The model under review builds one solid part; all positions refer to its coordinate system, in mm. Face numbers are marked on the shaded views. A direction names the side the tool comes from. Give positions to 0.01 mm unless a question says otherwise; leave off trailing zeros. Write each loop counter-clockwise with the first axis right and the second up, starting at its lowest first coordinate (ties: lowest second). Pieces come first, ordered by that corner, then holes.
from build123d import *

# Parameters (mm, degrees)
SKETCH1_W               = 101.6
SKETCH1_H               = 85.471
BOSS_EXTRUDE1_DEPTH     = 1.6002
SKETCH2_W               = 21.717
SKETCH2_H               = 16.002
ETHERNET_DEPTH          = 14.224
SKETCH3_W               = 13.9192
SKETCH3_H               = 8.89
POWER_CONNECTOR_DEPTH   = 10.6172
SKETCH4_W               = 9.0424
SKETCH4_H               = 32.9438
SKETCH4_H_2             = 20.2184
F_2X_CONNECTOR_DEPTH    = 9.2456
SKETCH6_W               = 15.24
SKETCH6_H               = 13.716
SD_CARD_DEPTH           = 2.3876
SKETCH7_R               = 5.08
CAPACATOR_DEPTH         = 16.9164
SKETCH5_R               = 1.6891
CORNER_HOLE_DEPTH       = 71.754645263
MIRROR2_COPY_1_SKETCH_R = 1.6891
MIRROR2_COPY_1_DEPTH    = 71.754645263


with BuildPart() as part:
    # Sketch1 → Boss-Extrude1 (new body)
    with BuildSketch(Plane.XY):
        Rectangle(SKETCH1_W, SKETCH1_H)
    extrude(amount=BOSS_EXTRUDE1_DEPTH)

    # Sketch2 → Ethernet (add)
    with BuildSketch(Plane.XY.offset(1.6002)):
        with Locations((-39.9415, 11.8745)):
            Rectangle(SKETCH2_W, SKETCH2_H)
    extrude(amount=ETHERNET_DEPTH)

    # Sketch3 → Power Connector (add)
    with BuildSketch(Plane.XY.offset(1.6002)):
        with Locations((-46.2534, -30.4165)):
            Rectangle(SKETCH3_W, SKETCH3_H)
    extrude(amount=POWER_CONNECTOR_DEPTH)

    # Sketch4 → 2x Connector (add)
    with BuildSketch(Plane.XY.offset(1.6002)):
        with Locations((48.7426, 12.954)):
            Rectangle(SKETCH4_W, SKETCH4_H)
        with Locations((48.7426, -13.6779)):
            Rectangle(SKETCH4_W, SKETCH4_H_2)
    extrude(amount=F_2X_CONNECTOR_DEPTH)

    # Sketch6 → SD Card (add)
    with BuildSketch(Plane.XY.offset(1.6002)):
        with Locations((-42.291, 28.8925)):
            Rectangle(SKETCH6_W, SKETCH6_H)
    extrude(amount=SD_CARD_DEPTH)

    # Sketch7 → Capacator (add)
    with BuildSketch(Plane.XY.offset(1.6002)):
        with Locations(Location((-26.797, -28.2575, 0), (0, 0, 180))):
            Circle(SKETCH7_R)
    extrude(amount=CAPACATOR_DEPTH)

    # Sketch5 → Corner Hole (cut, through all)
    with BuildSketch(Plane(origin=(0, 0, 0), x_dir=(-1, 0, 0), z_dir=(0, 0, -1))):
        with Locations((-47.3329, 39.4462)):
            Circle(SKETCH5_R)
    corner_hole = extrude(amount=-CORNER_HOLE_DEPTH, mode=Mode.SUBTRACT)

    # Mirror1: Corner Hole across plane
    add(corner_hole.mirror(Plane(origin=(0, 0, 0), x_dir=(0, 0, 1), z_dir=(1, 0, 0))), mode=Mode.SUBTRACT)

    # Mirror2: Corner Hole across plane
    add(corner_hole.mirror(Plane.ZX), mode=Mode.SUBTRACT)

    # Mirror2 copy 1 sketch → Mirror2 copy 1 (cut, through all)
    with BuildSketch(Plane(origin=(0, 0, 0), x_dir=(1, 0, 0), z_dir=(0, 0, -1))):
        with Locations((-47.3329, 39.4462)):
            Circle(MIRROR2_COPY_1_SKETCH_R)
    extrude(amount=-MIRROR2_COPY_1_DEPTH, mode=Mode.SUBTRACT)


solid = part.part
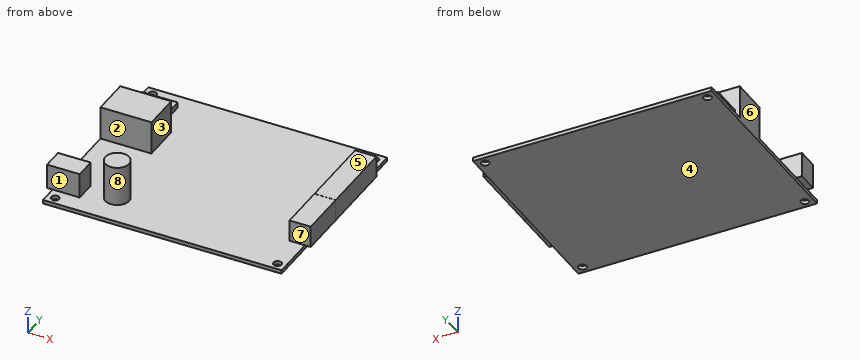
1) Consider section B-B, the plane y = -15. Give the boundary of the cut face in (x, z), then the cut area to 3 significant figures.
2) Consider section D-D, the plane y = 17. Give the boundary of the cut face in (x, z).
3) To check wall thickness, follow probe 1 along X at (y, z) = (9, 2.25); probe 2 along Y at (x, z) = (-43, 12); probe 3 along X at (y, z) = (-18, 9.5). State the ranges of each line that lie inside material, in increasing order.
4) Consider section A-A, the plane x = -38. Give the boundary of the cut face in (y, z).
5) Consider section C-C, the plane z = 9.5. Give the boundary of the cut face in (x, y).
6) The part is to be moulded in two halves that separate along X. For the marked faces 6, 7 and 8, say which applies: +X half, -X half, draft (parallel to the pull), parting line (faces both ways), or undercut.
7) Insertion check: pin 1 (1 mm diameter, centred on x = -8.5, y = -1, fed in from +Z); pin 2 (2.5 mm diameter, centred on y = 26.5, z = 2.5, fed in from -X); pin 3 (0.7 mm diameter, centred on x = -45, z = 2.5, fed in from +Y); pin 4 (4.5 mm diameter, centred on x = -47.33, y = -39.45, fed in from -Z). Each pin has a flat end and moves straight along its axis. Give the tip position at first contact, or say it passes through.
8) Tool access review of the marked faces 1, 2, 3, 4 and 5: name each direction out of +Z, -Z, +X, -X, +Y, -Y from which nothing blocks a thin tool from reaching the whole face with its end or side.
Answer block:
1. outline: (-50.8, 0) - (50.8, 0) - (50.8, 1.6) - (53.26, 1.6) - (53.26, 10.85) - (44.22, 10.85) - (44.22, 1.6) - (-50.8, 1.6) - close
1. area: 246 mm2
2. outline: (-50.8, 0) - (50.8, 0) - (50.8, 1.6) - (53.26, 1.6) - (53.26, 10.85) - (44.22, 10.85) - (44.22, 1.6) - (-29.08, 1.6) - (-29.08, 15.82) - (-50.8, 15.82) - close
3. probe 1: x = -50.8 to -29.08, 44.22 to 53.26
3. probe 2: y = -34.86 to -25.97, 3.87 to 19.88
3. probe 3: x = 44.22 to 53.26
4. outline: (-42.74, 0) - (42.74, 0) - (42.74, 1.6) - (35.75, 1.6) - (35.75, 3.99) - (22.03, 3.99) - (22.03, 1.6) - (19.88, 1.6) - (19.88, 15.82) - (3.87, 15.82) - (3.87, 1.6) - (-42.74, 1.6) - close
5. outline: (-53.21, -34.86) - (-39.29, -34.86) - (-39.29, -25.97) - (-53.21, -25.97) - close; (-50.8, 3.87) - (-29.08, 3.87) - (-29.08, 19.88) - (-50.8, 19.88) - close; circle Ø10.16 at (-26.8, -28.26); (44.22, -23.79) - (53.26, -23.79) - (53.26, -3.57) - (44.22, -3.57) - close; (44.22, -3.52) - (53.26, -3.52) - (53.26, 29.43) - (44.22, 29.43) - close
6. face 6: -X half
6. face 7: draft
6. face 8: undercut
7. pin 1: stops at z = 1.6
7. pin 2: stops at x = -50.8
7. pin 3: stops at y = 35.75
7. pin 4: stops at z = 0
8. face 1: +Z, +X, -X, -Y
8. face 2: +Z, -X
8. face 3: +Z, +Y
8. face 4: -Z, +X, -X, +Y, -Y
8. face 5: +Z, +X, +Y, -Y
